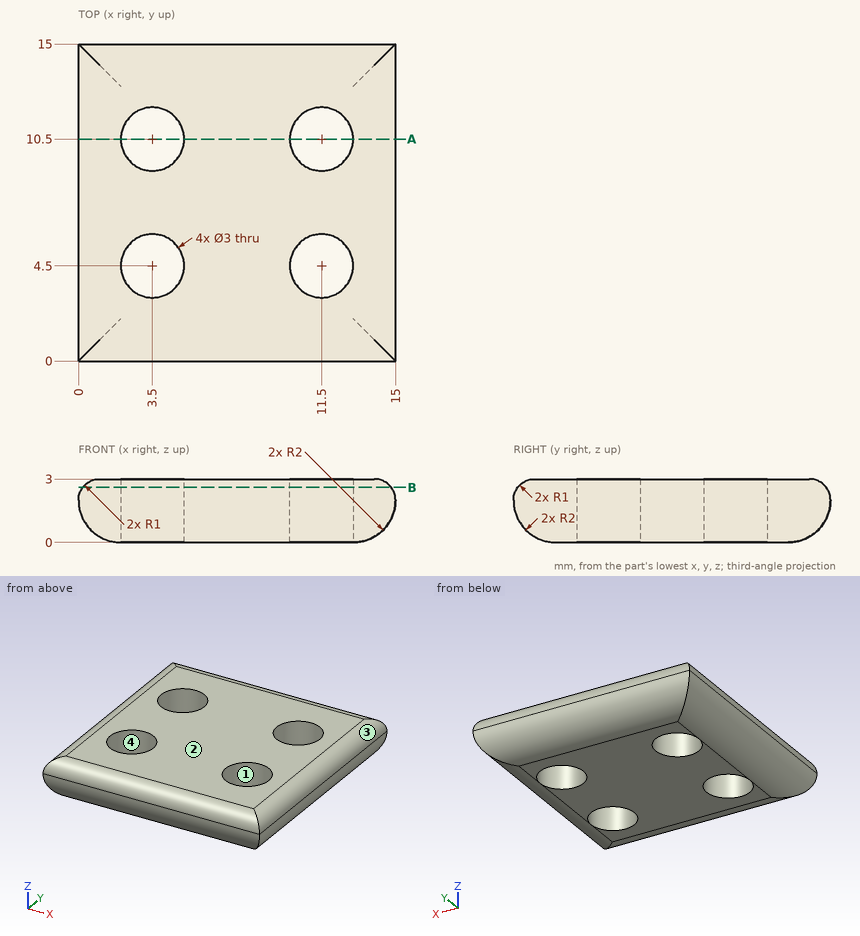
Geometry check sheet. Reference: drawing and pictorial views, mm from the part's lowest x, y, z. Round coordinates to 2 decimals unless told otherwise and drop trailing zeros. Order: outer loops, then holes, each group sorted by start corner. A loop starts at its lowest first (then second) coordinate and runs counter-clockwise, first axis right, second up. Notation, with made-up numbers: (18.25, 75) - (64.25, 75) arc R28 ccw to (64.25, 100) - close; hole circle Ø9 at (22, -0.75). An arc over 180 degrees is marked (long way). Use a Markdown table: item, result. Add a question column.
1) Mould release check, pull along X, two halves, no side actions. Record for the marked faces 1, 2, 3 and 4: released by +X, released by -X, zero draft, split by the parting line, or undercut.
2) Section check B-B (z = 2.6). Record the cut outline in (x, y), then the cut area to 3 significant figures.
3) Thickness scan on line 1 along Y through (x, z) = (3.5, 2.45); line 2 along Y through (x, z) = (3.25, 1.6); line 3 along X through (y, z) = (10.75, 2.1) (3 decimals). Record the ranges inside material, lowest first.
4) Section check A-A (y = 10.5). Count the separate pieces of the cut face and the enclosed holes in it.
Established:
| question | item | result |
|---|---|---|
| 1 | face 1 | undercut |
| 1 | face 2 | zero draft |
| 1 | face 3 | released by +X |
| 1 | face 4 | undercut |
| 2 | outline | (0.2, 0.2) - (14.8, 0.2) - (14.8, 14.8) - (0.2, 14.8) - close; hole circle Ø3 at (3.5, 4.5); hole circle Ø3 at (3.5, 10.5); hole circle Ø3 at (11.5, 4.5); hole circle Ø3 at (11.5, 10.5) |
| 2 | area | 185 mm2 |
| 3 | line 1 | 0.11 to 3, 6 to 9, 12 to 14.89 |
| 3 | line 2 | 0.04 to 3.02, 5.98 to 9.02, 11.98 to 14.96 |
| 3 | line 3 | 0.005 to 2.021, 4.979 to 10.021, 12.979 to 14.995 |
| 4 | separate pieces | 3 |
| 4 | enclosed holes | 0 |
